Print and shaded views of the part. All mm, measured from the part's lowest x, y and z. Round coordinates to 2 decimals unless told otherwise and drop trailing zeros. Order: outer loops, then holes, each group sorted by start corner. A loop starts at its lowest first (then second) coordinate and runs counter-clockwise, first axis right, second up. Notation, with made-up numbers: (-38, 38.25) - (-33, 38.25) arc R23 ccw to (-33, 58.25) - close; hole circle Ø5 at (12, 62.25). An arc over 180 degrees is marked (long way). Write item = value, one per line.
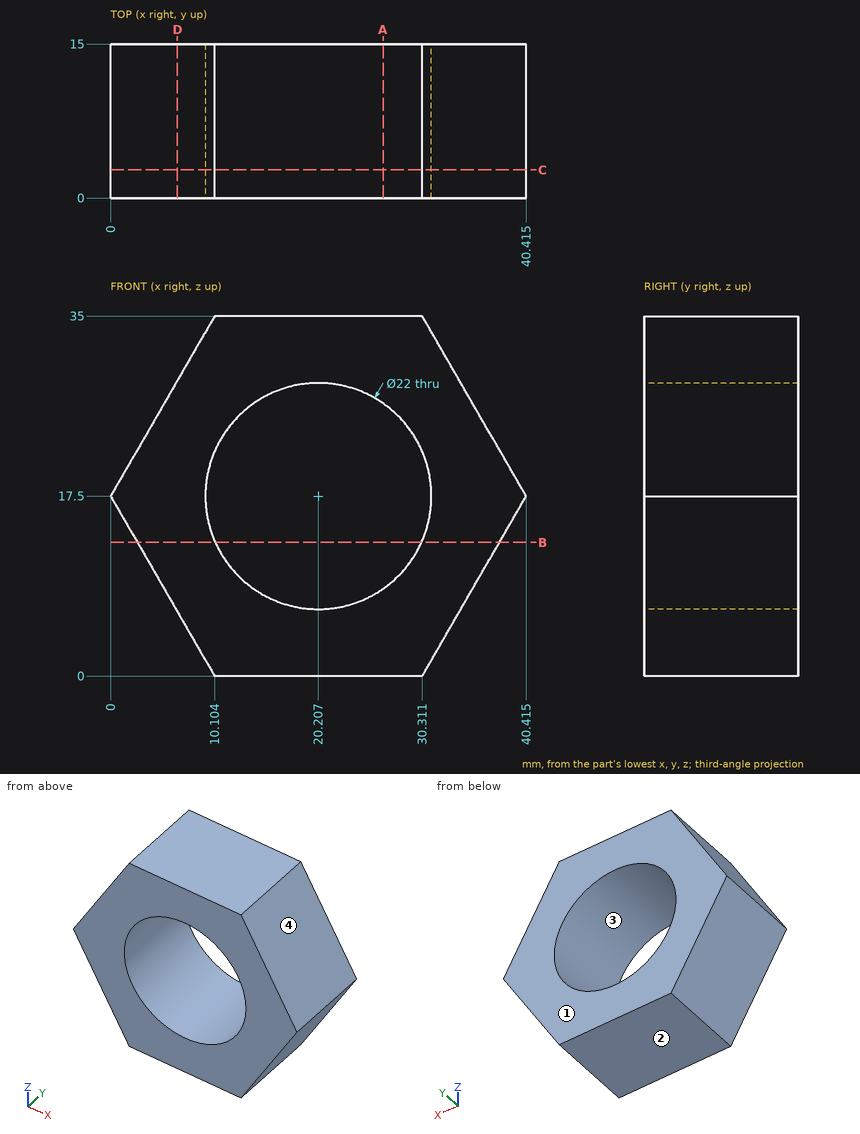
(1) Probe line 1 along X through (y, z) = (0.5, 20) (1 decimal); line 2 along Z through (x, y) = (30, 1.5); line 3 along Z through (x, y) = (23, 10). List the from-to ranges inside material, lowest first.
Solved:
line_1 = 1.4 to 9.5, 30.9 to 39
line_2 = 0 to 12.49, 22.51 to 35
line_3 = 0 to 6.86, 28.14 to 35
(2) Drop flat-ended pins along their axis: pin 1 (5 mm diameter, centred on y = 2.5, z = 13, fed in from -X) (1 decimal); pin 2 (5 mm diameter, centred on y = 9, z = 25.5, fed in from +X). Give the stop position or say it passes through.
Solved:
pin_1 = 1.2
pin_2 = 37.24
(3) Band-saw the part on B-B on z = 13. List the corners of the cut face in (x, y) (1 decimal).
Solved:
outline = (2.6, 0) - (10.2, 0) - (10.2, 15) - (2.6, 15) - close; (30.2, 0) - (37.8, 0) - (37.8, 15) - (30.2, 15) - close
(4) Pull direction Z, two halves, no side cores. Call the marked faces 1, 2, 3 and 4: released by +Z, released by -Z, zero draft, split by the parting line, or undercut.
Solved:
face_1 = zero draft
face_2 = released by -Z
face_3 = undercut
face_4 = released by +Z
(5) Band-saw the part on A-A on x = 26.5. List the corners of the cut face in (y, z).
Solved:
outline = (0, 0) - (15, 0) - (15, 8.48) - (0, 8.48) - close; (0, 26.52) - (15, 26.52) - (15, 35) - (0, 35) - close
(6) Band-saw the part on C-C on y = 2.75. List the corners of the cut face in (x, z) (1 decimal).
Solved:
outline = (0, 17.5) - (10.1, 0) - (30.3, 0) - (40.4, 17.5) - (30.3, 35) - (10.1, 35) - close; hole circle Ø22 at (20.2, 17.5)
(7) Band-saw the part on D-D on x = 6.5. List the corners of the cut face in (y, z).
Solved:
outline = (0, 6.24) - (15, 6.24) - (15, 28.76) - (0, 28.76) - close
